Here's how the part is built. I have some questions about the finished solid (model axes, mm). A direction names the side the tool comes from. Give positions to 0.01 mm unless a question says otherwise; leave off trailing zeros. Loops run counter-clockwise (first coordinate to the right, second up) from the corner with the lowest first, then second, coordinate; pieces in that order, holes last. Notation, with made-up numbers: (-1.75, -5.5) - (56.25, -5.5) arc R24 ccw to (56.25, 11.5) - close; hole circle Ø3 at (60, 16). An arc over 180 degrees is marked (long way). Use a Markdown table: item, result.
from build123d import *

# Parameters (mm, degrees)
SKETCH1_R           = 9.75
SKETCH1_R_2         = 1.65
BOSS_EXTRUDE1_DEPTH = 7
FILLET1_R           = 10
SKETCH2_R           = 9.75
SKETCH2_R_2         = 7.5
BOSS_EXTRUDE2_DEPTH = 2
SKETCH3_R           = 7.5
SKETCH3_R_2         = 3.5
BOSS_EXTRUDE3_DEPTH = 1.8
SKETCH4_W           = 1.8
SKETCH4_H           = 2.5
CUT_EXTRUDE1_DEPTH  = 2.5
SKETCH5_R           = 2.1
CUT_EXTRUDE2_DEPTH  = 3
SKETCH6_R           = 2.95
CUT_EXTRUDE3_DEPTH  = 3.2


with BuildPart() as part:
    # Sketch1 → Boss-Extrude1 (new body)
    with BuildSketch(Plane.XY):
        with BuildLine():
            Line((-35.5, 9.5), (-7.733854149, 9.5))
            ThreePointArc((-7.733854149, 9.5), (0, 12.25), (7.733854149, 9.5))
            Line((7.733854149, 9.5), (35.5, 9.5))
            ThreePointArc((35.5, 9.5), (38.681980515, 8.181980515), (40, 5))
            Line((40, 5), (40, -11))
            ThreePointArc((40, -11), (38.681980515, -14.181980515), (35.5, -15.5))
            Line((35.5, -15.5), (-35.5, -15.5))
            ThreePointArc((-35.5, -15.5), (-38.681980515, -14.181980515), (-40, -11))
            Line((-40, -11), (-40, 5))
            ThreePointArc((-40, 5), (-38.681980515, 8.181980515), (-35.5, 9.5))
        make_face()
        Circle(SKETCH1_R, mode=Mode.SUBTRACT)
        with Locations((-35.5, 5)):
            Circle(SKETCH1_R_2, mode=Mode.SUBTRACT)
        with Locations((35.5, 5)):
            Circle(SKETCH1_R_2, mode=Mode.SUBTRACT)
        with Locations((-35.5, -11)):
            Circle(SKETCH1_R_2, mode=Mode.SUBTRACT)
        with Locations((35.5, -11)):
            Circle(SKETCH1_R_2, mode=Mode.SUBTRACT)
    extrude(amount=BOSS_EXTRUDE1_DEPTH)

    # Fillet1
    fillet1_edges = [part.edges().sort_by_distance(p)[0] for p in [
        (7.733854149, 9.5, 3.5),
        (-7.733854149, 9.5, 3.5),
    ]]
    fillet(fillet1_edges, radius=FILLET1_R)

    # Sketch2 → Boss-Extrude2 (add)
    with BuildSketch(Plane.XY.offset(7)):
        Circle(SKETCH2_R)
        Circle(SKETCH2_R_2, mode=Mode.SUBTRACT)
    extrude(amount=-BOSS_EXTRUDE2_DEPTH)

    # Sketch3 → Boss-Extrude3 (add)
    with BuildSketch(Plane.XY.offset(7)):
        Circle(SKETCH3_R)
        Circle(SKETCH3_R_2, mode=Mode.SUBTRACT)
    extrude(amount=-BOSS_EXTRUDE3_DEPTH)

    # Sketch4 → Cut-Extrude1 (cut)
    with BuildSketch(Plane.XY.offset(7)):
        with Locations((8, 0)):
            Rectangle(SKETCH4_W, SKETCH4_H)
    extrude(amount=-CUT_EXTRUDE1_DEPTH, mode=Mode.SUBTRACT)

    # Sketch5 → Cut-Extrude2 (cut)
    with BuildSketch(Plane.XY.offset(7)):
        with Locations((-14, 0)):
            Circle(SKETCH5_R)
        with Locations((14, 0)):
            Circle(SKETCH5_R)
    extrude(amount=-CUT_EXTRUDE2_DEPTH, mode=Mode.SUBTRACT)

    # Sketch6 → Cut-Extrude3 (cut)
    with BuildSketch(Plane.XY.offset(7)):
        with Locations((-35.5, 5)):
            Circle(SKETCH6_R)
        with Locations((-35.5, -11)):
            Circle(SKETCH6_R)
        with Locations((35.5, -11)):
            Circle(SKETCH6_R)
        with Locations((35.5, 5)):
            Circle(SKETCH6_R)
    extrude(amount=-CUT_EXTRUDE3_DEPTH, mode=Mode.SUBTRACT)


solid = part.part
(1) Suppose I cut it at B-B on y = 0. Write out the boundary of the cut face in (x, z).
A:
| item | result |
|---|---|
| outline | (-40, 0) - (-9.75, 0) - (-9.75, 5) - (-7.5, 5) - (-7.5, 5.2) - (-3.5, 5.2) - (-3.5, 7) - (-11.9, 7) - (-11.9, 4) - (-16.1, 4) - (-16.1, 7) - (-40, 7) - close; (3.5, 5.2) - (7.1, 5.2) - (7.1, 7) - (3.5, 7) - close; (8.9, 5) - (9.75, 5) - (9.75, 0) - (40, 0) - (40, 7) - (16.1, 7) - (16.1, 4) - (11.9, 4) - (11.9, 7) - (8.9, 7) - close |
(2) Suppose I cut it at D-D on x = 14. Write out the boundary of the cut face in (y, z), plus the area to 3 significant figures.
A:
| item | result |
|---|---|
| outline | (-15.5, 0) - (9.5, 0) - (9.5, 7) - (2.1, 7) - (2.1, 4) - (-2.1, 4) - (-2.1, 7) - (-15.5, 7) - close |
| area | 162 mm2 |
(3) Will these pins go through, and if not, where does the flat tip stop? pin 1 (3 mm diameter, centred on x = 36, y = -12.5, fed in from +Z); pin 2 (5.5 mm diameter, centred on x = -35.5, y = -11, fed in from +Z); pin 3 (2 mm diameter, centred on x = 31, z = 5, fed in from +Y); pin 4 (1.4 mm diameter, centred on x = 7.5, z = 5.5, fed in from +Y).
A:
| item | result |
|---|---|
| pin 1 | z = 7 |
| pin 2 | z = 3.8 |
| pin 3 | y = 9.5 |
| pin 4 | y = 10.3 |
(4) Suppose I cut it at A-A on x = 0. Write out the boundary of the cut face in (y, z), plus the area to 4 significant figures.
A:
| item | result |
|---|---|
| outline | (-15.5, 0) - (-9.75, 0) - (-9.75, 5) - (-7.5, 5) - (-7.5, 5.2) - (-3.5, 5.2) - (-3.5, 7) - (-15.5, 7) - close; (3.5, 5.2) - (7.5, 5.2) - (7.5, 5) - (9.75, 5) - (9.75, 0) - (12.25, 0) - (12.25, 7) - (3.5, 7) - close |
| area | 81.15 mm2 |
(5) On a 3-axis mill with a long thin cutter (end or side, diameter ignored), from which of +Z, -Z, +X, -X, +Y, -Y can I reach the whole of each face in a straight line? I mean faces 1 (the face through (-1.269, 9.667, 2.465)), 2 (the face through (7.1, 0, 6)), 3 (the face through (37.086, -8.513, 5.422)). Say none if no direction works.
A:
| item | result |
|---|---|
| face 1 | -Z |
| face 2 | +Z, -Z |
| face 3 | +Z |
(6) We'd pull the mould along Y, two halves only. Please class faces 4 (the face through (-38.647, -14.217, 3.451)), 5 (the face through (-23, 9.5, 3)), 6 (the face through (37, 4, 3.8)): pulls with the +Y half, pulls with the -Y half, needs draft (parallel to the pull), parting line crosses it, or undercut.
A:
| item | result |
|---|---|
| face 4 | pulls with the -Y half |
| face 5 | pulls with the +Y half |
| face 6 | undercut |
(7) If I drill on line 1 (X direction, y = -11, z = 2.85); line 2 (Y direction, x = 35.5, z = 4.8); line 3 (Y direction, x = -35.5, z = 1.75), over which ranges is the centre line in solid material (lowest first)?
A:
| item | result |
|---|---|
| line 1 | -40 to -37.15, -33.85 to 33.85, 37.15 to 40 |
| line 2 | -15.5 to -13.95, -8.05 to 2.05, 7.95 to 9.5 |
| line 3 | -15.5 to -12.65, -9.35 to 3.35, 6.65 to 9.5 |
(8) Suppose I cut it at C-C on z = 1.75. Write out the boundary of the cut face in (x, y).
A:
| item | result |
|---|---|
| outline | (-40, -11) arc R4.5 ccw to (-35.5, -15.5) - (35.5, -15.5) arc R4.5 ccw to (40, -11) - (40, 5) arc R4.5 ccw to (35.5, 9.5) - (10.72, 9.5) arc R10 cw to (5.9, 10.74) arc R12.25 ccw to (-5.9, 10.74) arc R10 cw to (-10.72, 9.5) - (-35.5, 9.5) arc R4.5 ccw to (-40, 5) - close; hole circle Ø3.3 at (-35.5, -11); hole circle Ø3.3 at (-35.5, 5); hole circle Ø19.5 at (0, 0); hole circle Ø3.3 at (35.5, -11); hole circle Ø3.3 at (35.5, 5) |
